```python
from build123d import *

# Parameters (mm, degrees)
F0_R     = 3.175
F1_DEPTH = 1.70815


with BuildPart() as f1:
    # F0 (on Top) → F1 (new body, symmetric)
    with BuildSketch(Plane.XY):
        with BuildLine():
            ThreePointArc((16.51, 25.4), (14.650128, 29.890128), (10.16, 31.75))
            Line((10.16, 31.75), (-10.16, 31.75))
            ThreePointArc((-10.16, 31.75), (-14.650128, 29.890128), (-16.51, 25.4))
            Line((-16.51, 25.4), (-16.51, -25.4))
            ThreePointArc((-16.51, -25.4), (-14.650128, -29.890128), (-10.16, -31.75))
            Line((-10.16, -31.75), (10.16, -31.75))
            ThreePointArc((10.16, -31.75), (14.650128, -29.890128), (16.51, -25.4))
            Line((16.51, -25.4), (16.51, 25.4))
        make_face()
        with Locations((-10.16, -25.4)):
            Circle(F0_R, mode=Mode.SUBTRACT)
        with Locations((10.16, -25.4)):
            Circle(F0_R, mode=Mode.SUBTRACT)
        with Locations((-10.16, 25.4)):
            Circle(F0_R, mode=Mode.SUBTRACT)
        with BuildLine():
            Line((-6.4135, 3.302), (6.4135, 3.302))
            ThreePointArc((6.4135, 3.302), (6.638006, 3.209006), (6.731, 2.9845))
            Line((6.731, 2.9845), (6.731, -2.9845))
            ThreePointArc((6.731, -2.9845), (6.638006, -3.209006), (6.4135, -3.302))
            Line((6.4135, -3.302), (-6.4135, -3.302))
            ThreePointArc((-6.4135, -3.302), (-6.638006, -3.209006), (-6.731, -2.9845))
            Line((-6.731, -2.9845), (-6.731, 2.9845))
            ThreePointArc((-6.731, 2.9845), (-6.638006, 3.209006), (-6.4135, 3.302))
        make_face(mode=Mode.SUBTRACT)
        with Locations((10.16, 25.4)):
            Circle(F0_R, mode=Mode.SUBTRACT)
    extrude(amount=F1_DEPTH, both=True)


solid = f1.part
```
Design review of the part built by this model. Coordinates are the model's own, in mm. A direction names the side the tool comes from. Give positions to 0.01 mm unless a question says otherwise; leave off trailing zeros. Order: outer loops, then holes, each group sorted by start corner. A loop starts at its lowest first (then second) coordinate and runs counter-clockwise, first axis right, second up. Notation, with made-up numbers: (26.5, 5) -> (63.5, 5) arc R17 cw to (63.5, 36) -> close; hole circle Ø2 at (35, 45). An arc over 180 degrees is marked (long way). Write each question's results on one line, items separated by ' | '. Start each with the question number.
Q1. For pin 1 (10 mm diameter, centred on x = -10.16, y = 25.4, fed in from +Z), flat-tipped, find the tip position at first contact; note if it passes through.
Q2. Machinability: for faces 5 (the flat face through (0, 3.302, 0)), 6 (the flat face through (0, 8, 1.708)), which of the approach directions +Z, -Z, +X, -X, +Y, -Y give a long, thin tool a straight path to every point of the face, cutting with its end or side? Answer none if there is none.
Q3. Add section C-C on x = 11. Give the boundary of the cut face in (y, z).
Q4. Wall thickness on L1, parallel to Y at x = -10.16, z = 0 (3 decimals); L2, parallel to Y at x = -6, z = 0.1; L3, parallel to Y at x = -7.5, z = -1.55: over which ranges is each line inside the solid? List them lowest first. Write a range as from..to.
Q5. Mouldability with a two-part tool opening along Y and no side actions: class faces 1 (the cylindrical face through (14.6, -29.94, 0.02)), 2 (the flat face through (0, 8, -1.708)), 3 (the cylindrical face through (9.75, 28.55, -0.02)), 4 (the cylindrical face through (14.7, 29.84, 0.02)) as +Y half, -Y half, draft (parallel to the pull), parting line (faces both ways), or undercut.
Q6. Add section A-A on z = -0.75. State how many separate pieces and enclosed holes the cut face has, and give its area (3 significant figures).
Q7. Add section B-B on x = 1.5. Give the boundary of the cut face in (y, z).
Found:
1) pin 1: stops at z = 1.71
2) face 5: +Z, -Z | face 6: +Z, +X, -X, +Y, -Y
3) outline: (-31.69, -1.71) -> (-28.46, -1.71) -> (-28.46, 1.71) -> (-31.69, 1.71) -> close; (-22.34, -1.71) -> (22.34, -1.71) -> (22.34, 1.71) -> (-22.34, 1.71) -> close; (28.46, -1.71) -> (31.69, -1.71) -> (31.69, 1.71) -> (28.46, 1.71) -> close
4) L1: y = -31.75..-28.575, -22.225..22.225, 28.575..31.75 | L2: y = -31.75..-3.3, 3.3..31.75 | L3: y = -31.75..-27.13, -23.67..23.67, 27.13..31.75
5) face 1: -Y half | face 2: draft | face 3: undercut | face 4: +Y half
6) separate pieces: 1 | enclosed holes: 5 | area: 1,850 mm2
7) outline: (-31.75, -1.71) -> (-3.3, -1.71) -> (-3.3, 1.71) -> (-31.75, 1.71) -> close; (3.3, -1.71) -> (31.75, -1.71) -> (31.75, 1.71) -> (3.3, 1.71) -> close
